```python
from build123d import *

# Parameters (mm, degrees)
CROQUIS1_R              = 75
SALIENTE_EXTRUIR1_DEPTH = 5
CROQUIS2_R              = 1.5
CORTAR_EXTRUIR1_DEPTH   = 5
CROQUIS3_R              = 1.5
CORTAR_EXTRUIR2_DEPTH   = 5


with BuildPart() as part:
    # Croquis1 → Saliente-Extruir1 (new body)
    with BuildSketch(Plane(origin=(0, 0, 0), x_dir=(1, 0, 0), z_dir=(0, 1, 0))):
        with Locations(Location((0, 0, 0), (0, 0, 270))):
            Circle(CROQUIS1_R)
    extrude(amount=SALIENTE_EXTRUIR1_DEPTH)

    # Croquis2 → Cortar-Extruir1 (cut)
    with BuildSketch(Plane(origin=(0, 5, 0), x_dir=(1, 0, 0), z_dir=(0, 1, 0))):
        with Locations(Location((0, 0, 0), (0, 0, 270))):
            Circle(CROQUIS2_R)
        with Locations(Location((7, 0, 0), (0, 0, 270))):
            Circle(CROQUIS2_R)
        with Locations(Location((0, -7, 0), (0, 0, 270))):
            Circle(CROQUIS2_R)
        with Locations(Location((-7, 0, 0), (0, 0, 270))):
            Circle(CROQUIS2_R)
        with Locations(Location((0, 7, 0), (0, 0, 270))):
            Circle(CROQUIS2_R)
    extrude(amount=-CORTAR_EXTRUIR1_DEPTH, mode=Mode.SUBTRACT)

    # Croquis3 → Cortar-Extruir2 (cut)
    with BuildSketch(Plane(origin=(0, 5, 0), x_dir=(1, 0, 0), z_dir=(0, 1, 0))):
        with BuildLine():
            ThreePointArc((28.5, 30), (28.939339828, 28.939339828), (30, 28.5))
            Line((30, 28.5), (30, 30))
            Line((30, 30), (28.5, 30))
        make_face()
        with BuildLine():
            Line((30, 30), (30, 28.5))
            ThreePointArc((30, 28.5), (31.060660172, 28.939339828), (31.5, 30))
            ThreePointArc((31.5, 30), (30, 31.5), (28.5, 30))
            Line((28.5, 30), (30, 30))
        make_face()
        with BuildLine():
            Line((-30, -28.5), (-30, -30))
            Line((-30, -30), (-28.5, -30))
            ThreePointArc((-28.5, -30), (-28.939339828, -28.939339828), (-30, -28.5))
        make_face()
        with BuildLine():
            Line((-28.5, -30), (-30, -30))
            Line((-30, -30), (-30, -28.5))
            ThreePointArc((-30, -28.5), (-31.060660172, -31.060660172), (-28.5, -30))
        make_face()
        with BuildLine():
            ThreePointArc((30, -28.5), (28.939339828, -28.939339828), (28.5, -30))
            Line((28.5, -30), (30, -30))
            Line((30, -30), (30, -28.5))
        make_face()
        with BuildLine():
            Line((30, -30), (28.5, -30))
            ThreePointArc((28.5, -30), (30, -31.5), (31.5, -30))
            ThreePointArc((31.5, -30), (31.060660172, -28.939339828), (30, -28.5))
            Line((30, -28.5), (30, -30))
        make_face()
        with Locations(Location((-30, 30, 0), (0, 0, 270))):
            Circle(CROQUIS3_R)
    extrude(amount=-CORTAR_EXTRUIR2_DEPTH, mode=Mode.SUBTRACT)


solid = part.part
```
Geometry: final body of the model. Coordinates: model frame, mm. Round coordinates to 2 decimals unless told otherwise and drop trailing zeros. Write each loop counter-clockwise with the first axis right and the second up, starting at its lowest first coordinate (ties: lowest second). Pieces come first, ordered by that corner, then holes.
Item 1: Material intervals for L1, parallel to X at y = 3.95, z = 0; L2, parallel to X at y = 4.75, z = -1; L3, parallel to X at y = 0.2, z = 6.5, sorted ascending.
Item 2: Pin query (flat end, axial travel): P1, Ø2.5, axis at x = -30, z = 30, coming from the +Y side; P2, Ø2, axis at x = 30.5, y = 1, coming from the -Z side; P3, Ø1, axis at x = 3, y = 2.5, coming from the -Z side; P4, Ø3, axis at x = 26, y = 2.5, coming from the +Z side. Return the tip coordinate at first contact, or that it passes through.
Item 3: Section query A-A (y = 3.2). Give the number of separate pieces and of enclosed holes in the cut face, plus the area to 3 significant figures.
Item 4: Section query C-C (z = -62). Return loops of the section in (x, y).
Item 5: Section query B-B (x = -17). Return loops of the section in (y, z).
Completed:
1. L1: x = -75 to -8.5, -5.5 to -1.5, 1.5 to 5.5, 8.5 to 75
1. L2: x = -74.99 to -8.12, -5.88 to -1.12, 1.12 to 5.88, 8.12 to 74.99
1. L3: x = -74.72 to -1.41, 1.41 to 74.72
2. P1: passes through
2. P2: stops at z = -68.95
2. P3: stops at z = -74.96
2. P4: stops at z = 70.89
3. separate pieces: 1
3. enclosed holes: 9
3. area: 17,600 mm2
4. outline: (-42.2, 0) - (42.2, 0) - (42.2, 5) - (-42.2, 5) - close
5. outline: (0, -73.05) - (5, -73.05) - (5, 73.05) - (0, 73.05) - close
